Autodesk Inventor part; units mm, degrees
ref_plane "YZ Plane" through (0, 0, 0) normal (1, 0, 0) x (0, 1, 0)
ref_plane "XZ Plane" through (0, 0, 0) normal (0, 1, 0) x (-1, 0, 0)
ref_plane "XY Plane" through (0, 0, 0) normal (0, 0, 1) x (1, 0, 0)
sketch "스케치1" plane through (0, 0, 0) normal (0, 1, 0) x (-1, 0, 0)
  line L0 (-24.9446, -24.9446) -> (24.9446, -24.9446)
  line L1 (24.9446, -24.9446) -> (24.9446, 24.9446)
  line L2 (24.9446, 24.9446) -> (-24.9446, 24.9446)
  line L3 (-24.9446, 24.9446) -> (-24.9446, -24.9446)
  line L4 (-24.9446, -24.9446) -> (24.9446, 24.9446) construction
  line L5 (24.9446, -24.9446) -> (-24.9446, 24.9446) construction
  line L6 (-28.1446, -28.1446) -> (28.1446, -28.1446)
  line L7 (28.1446, -28.1446) -> (28.1446, 28.1446)
  line L8 (28.1446, 28.1446) -> (-28.1446, 28.1446)
  line L9 (-28.1446, 28.1446) -> (-28.1446, -28.1446)
  line L10 (-28.1446, -28.1446) -> (28.1446, 28.1446) construction
  line L11 (28.1446, -28.1446) -> (-28.1446, 28.1446) construction
  point P0 (0, 0)
  dimension "d0" = 70.554
  dimension "d1" = 3.2
extrude "돌출1" add sketch "스케치1" along normal blind 3.7 contours L3 L2 L1 L0 | L9 L8 L7 L6
sketch "스케치2" plane through (0, 3.7, 0) normal (0, 1, 0) x (1, 0, 0)
  line L0 (-28.1446, 28.1446) -> (-28.1446, -28.1446)
  line L1 (-28.1446, -28.1446) -> (28.1446, -28.1446)
  line L2 (28.1446, -28.1446) -> (28.1446, 28.1446)
  line L3 (28.1446, 28.1446) -> (-28.1446, 28.1446)
  line L4 (26.5446, 26.5446) -> (-26.5446, 26.5446)
  line L5 (-26.5446, 26.5446) -> (-26.5446, -26.5446)
  line L6 (-26.5446, -26.5446) -> (26.5446, -26.5446)
  line L7 (26.5446, -26.5446) -> (26.5446, 26.5446)
  line L8 (26.5446, 26.5446) -> (-26.5446, -26.5446) construction
  line L9 (-26.5446, 26.5446) -> (26.5446, -26.5446) construction
  line L10 (24.5446, 24.5446) -> (-24.5446, 24.5446)
  line L11 (-24.5446, 24.5446) -> (-24.5446, -24.5446)
  line L12 (-24.5446, -24.5446) -> (24.5446, -24.5446)
  line L13 (24.5446, -24.5446) -> (24.5446, 24.5446)
  line L14 (24.5446, 24.5446) -> (-24.5446, -24.5446) construction
  line L15 (-24.5446, 24.5446) -> (24.5446, -24.5446) construction
  point P0 (0, 0)
  point P1 (0, 28.1446)
  point P2 (-28.1446, 0)
  dimension "d4" = 1.6
  dimension "d5" = 2
extrude "돌출2" cut sketch "스케치2" against normal blind 1.2 contours L7 L6 L5 L4 | L13 L12 L11 L10
sketch "스케치3" plane through (0, 2.5, 0) normal (0, 1, 0) x (1, 0, 0)
  line L0 (24.5446, 24.5446) -> (-24.5446, 24.5446)
  line L1 (-24.5446, 24.5446) -> (-24.5446, -24.5446)
  line L2 (-24.5446, -24.5446) -> (24.5446, -24.5446)
  line L3 (24.5446, -24.5446) -> (24.5446, 24.5446)
  line L4 (24.5446, 24.5446) -> (-24.5446, -24.5446) construction
  line L5 (-24.5446, 24.5446) -> (24.5446, -24.5446) construction
  line L6 (-26.5446, -26.5446) -> (-26.5446, 26.5446)
  point P0 (0, 0)
  dimension "d8" = 2
extrude "돌출3" add sketch "스케치3" along normal blind 0.6
fillet "모깎기1" radius 1.2 8 edges at (0, 3.7, 28.1446) (28.1446, 3.7, 0) (0, 3.7, -28.1446) (-28.1446, 3.7, 0) (-28.1446, 0, 0) (0, 0, 28.1446) (28.1446, 0, 0) (0, 0, -28.1446)
sketch "스케치10" plane through (0, 0, 0) normal (0, -1, 0) x (1, 0, 0)
  line L0 (-12.5, 10.3) -> (12.5, 10.3)
  line L1 (12.5, 10.3) -> (12.5, 15.3)
  line L2 (12.5, 15.3) -> (-12.5, 15.3)
  line L3 (-12.5, 15.3) -> (-12.5, 10.3)
  line L4 (-12.5, 10.3) -> (12.5, 15.3) construction
  line L5 (12.5, 10.3) -> (-12.5, 15.3) construction
  line L6 (0, 0) -> (6.1954, 0)
  line L7 (-12.5, -10.3) -> (12.5, -10.3)
  line L8 (12.5, -10.3) -> (12.5, -15.3)
  line L9 (12.5, -15.3) -> (-12.5, -15.3)
  line L10 (-12.5, -15.3) -> (-12.5, -10.3)
  line L11 (-12.5, -10.3) -> (12.5, -15.3) construction
  line L12 (12.5, -10.3) -> (-12.5, -15.3) construction
  point P0 (0, 12.8)
  point P1 (0, -12.8)
  dimension "d51" = 25
  dimension "d52" = 5
  dimension "d53" = 10.3
extrude "돌출7" add sketch "스케치10" along normal blind 15
sketch "스케치11" plane through (12.5, 0, -15.3) normal (0, 0, -1) x (-1, 0, 0)
  circle A0 centre (17.5, -7.5) radius 1.25
  line L0 (-14.4446, 0) -> (39.4446, 0)
  line L1 (12.5, 0) -> (12.5, -4.6677)
  circle A1 centre (7.5, -7.5) radius 1.25
  dimension "d56" = 2.5
  dimension "d57" = 7.5
  dimension "d58" = 5
extrude "돌출8" cut sketch "스케치11" against normal up to surface (30.6 mm away)
equation "\"d39\" = 55deg"
properties part number "OV-PAM_n_4_bottom"
For this review, take the finished solid that the model builds, in its own axes (mm). A direction names the side the tool comes from. Round coordinates to 2 decimals unless told otherwise and drop trailing zeros. Loops run counter-clockwise (first coordinate to the right, second up) from the corner with the lowest first, then second, coordinate; pieces in that order, holes last. Notation, with made-up numbers: (47, -8.75) - (90, -8.75) arc R17 ccw to (90, -3.75) - close; hole circle Ø10 at (-32, 20). An arc over 180 degrees is marked (long way). Use one line per item in the form item = value.
Item 1: Consider section B-B on y = -12. Write out the cut boundary in (x, z).
Answers:
outline = (-12.5, -15.3) - (12.5, -15.3) - (12.5, -10.3) - (-12.5, -10.3) - close; (-12.5, 10.3) - (12.5, 10.3) - (12.5, 15.3) - (-12.5, 15.3) - close
Item 2: Consider section D-D on y = -7.5. Write out the cut boundary in (x, z).
Answers:
outline = (-12.5, -15.3) - (-6.25, -15.3) - (-6.25, -10.3) - (-12.5, -10.3) - close; (-12.5, 10.3) - (-6.25, 10.3) - (-6.25, 15.3) - (-12.5, 15.3) - close; (-3.75, -15.3) - (3.75, -15.3) - (3.75, -10.3) - (-3.75, -10.3) - close; (-3.75, 10.3) - (3.75, 10.3) - (3.75, 15.3) - (-3.75, 15.3) - close; (6.25, -15.3) - (12.5, -15.3) - (12.5, -10.3) - (6.25, -10.3) - close; (6.25, 10.3) - (12.5, 10.3) - (12.5, 15.3) - (6.25, 15.3) - close
Item 3: Mouldability with a two-part tool opening along Z and no side actions: class faces 1 (the flat face through (0, 2, -28.145)), 2 (the flat face through (0, -7, 10.3)), 3 (the flat face through (-12.5, -7, 13)) as +Z half, -Z half, draft (parallel to the pull), parting line (faces both ways), or undercut.
Answers:
face_1 = -Z half
face_2 = undercut
face_3 = draft
Item 4: For line 1 (Y direction, x = 5, z = 12); line 2 (Z direction, x = -4, y = -13.5); line 3 (X direction, y = 3, z = 15), list the stretches that pass through material, from the lowest coordinate up.
Answers:
line_1 = -15 to -8.75, -6.25 to 3.1
line_2 = -15.3 to -10.3, 10.3 to 15.3
line_3 = -28.04 to -26.54, -24.54 to 24.54, 26.54 to 28.04
Item 5: Consider section A-A on x = 5. State how many separate pieces and enclosed holes the cut face has, then the cut area to 3 significant figures.
Answers:
separate_pieces = 3
enclosed_holes = 0
area = 298 mm^2
Item 6: Consider section C-C on z = 14. Write out the cut boundary in (x, y), then the cut area to 3 significant figures.
Answers:
outline = (-28.14, 1.2) arc R1.2 ccw to (-26.94, 0) - (-12.5, 0) - (-12.5, -15) - (12.5, -15) - (12.5, 0) - (26.94, 0) arc R1.2 ccw to (28.14, 1.2) - (28.14, 2.5) arc R1.2 ccw to (26.94, 3.7) - (26.54, 3.7) - (26.54, 2.5) - (24.54, 2.5) - (24.54, 3.1) - (-24.54, 3.1) - (-24.54, 2.5) - (-26.54, 2.5) - (-26.54, 3.7) - (-26.94, 3.7) arc R1.2 ccw to (-28.14, 2.5) - close; hole circle Ø2.5 at (-5, -7.5); hole circle Ø2.5 at (5, -7.5)
area = 538 mm^2
Item 7: Clearance check with flat-ended pins moving along their axes: P1, Ø1.5, axis at x = -4.5, y = -4.5, coming from the -Z side; P2, Ø8, axis at x = 10, z = 8, coming from the +Y side; P3, Ø1.5, axis at y = -5.5, z = -12.5, coming from the +X side. State where each tip first meets the part, or that it passes through.
Answers:
P1 = -15.3
P2 = 3.1
P3 = 12.5
Item 8: Tool access review of faces 4 (the flat face through (-12.5, -7, -13)), 5 (the flat face through (0, -7, -10.3)), 6 (the flat face through (0, -7, -15.3)), 7 (the flat face through (12.5, -7, 13)), 8 (the flat face through (0, -7, 15.3)): name each direction out of +Z, -Z, +X, -X, +Y, -Y from which nothing blocks a thin tool from reaching the whole face with its end or side.
Answers:
face_4 = +Z, -Z, -X, -Y
face_5 = +X, -X, -Y
face_6 = -Z, +X, -X, -Y
face_7 = +Z, -Z, +X, -Y
face_8 = +Z, +X, -X, -Y
